from build123d import *

# Parameters (mm, degrees)
SKETCH1_W           = 56.15
SKETCH1_H           = 25.4
BOSS_EXTRUDE1_DEPTH = 2.54
SKETCH2_W           = 56.15
SKETCH2_H           = 25.4
BOSS_EXTRUDE2_DEPTH = 2.54
SKETCH11_W          = 56.15
SKETCH11_H          = 25.4
BOSS_EXTRUDE3_DEPTH = 5.715
SKETCH6_R           = 1.774
CUT_EXTRUDE3_DEPTH  = 9.255
SKETCH13_W          = 56.15
SKETCH13_H          = 31.115
BOSS_EXTRUDE4_DEPTH = 11.938
SKETCH14_W          = 12.7
SKETCH14_H          = 8.89
SKETCH14_W_2        = 33.02
CUT_EXTRUDE4_DEPTH  = 32.115
SKETCH17_W          = 10.43
SKETCH17_H          = 22.86
BOSS_EXTRUDE5_DEPTH = 14.097
SKETCH15_R          = 1.778
CUT_EXTRUDE5_DEPTH  = 38.338


with BuildPart() as part:
    # Sketch1 → Boss-Extrude1 (new body)
    with BuildSketch(Plane(origin=(0, 0, 0), x_dir=(1, 0, 0), z_dir=(0, 1, 0))):
        with Locations((28.075, 12.7)):
            Rectangle(SKETCH1_W, SKETCH1_H)
    extrude(amount=-BOSS_EXTRUDE1_DEPTH)

    # Sketch2 → Boss-Extrude2 (add)
    with BuildSketch(Plane.XY):
        with Locations((28.075, -12.7)):
            Rectangle(SKETCH2_W, SKETCH2_H)
    extrude(amount=-BOSS_EXTRUDE2_DEPTH)

    # Sketch11 → Boss-Extrude3 (add)
    with BuildSketch(Plane(origin=(0, 0, 0), x_dir=(1, 0, 0), z_dir=(0, 1, 0))):
        with Locations((28.075, 12.7)):
            Rectangle(SKETCH11_W, SKETCH11_H)
    extrude(amount=BOSS_EXTRUDE3_DEPTH)

    # Sketch6 → Cut-Extrude3 (cut, through all)
    with BuildSketch(Plane.XZ.offset(2.54)):
        with Locations((52.852, -22.102)):
            Circle(SKETCH6_R)
        with Locations((52.852, -9.664)):
            Circle(SKETCH6_R)
        with Locations((3.298, -9.664)):
            Circle(SKETCH6_R)
        with Locations((3.298, -22.102)):
            Circle(SKETCH6_R)
    extrude(amount=-CUT_EXTRUDE3_DEPTH, mode=Mode.SUBTRACT)

    # Sketch13 → Boss-Extrude4 (add)
    with BuildSketch(Plane.XY):
        with Locations((28.075, -9.8425)):
            Rectangle(SKETCH13_W, SKETCH13_H)
    extrude(amount=BOSS_EXTRUDE4_DEPTH)

    # Sketch14 → Cut-Extrude4 (cut, through all)
    with BuildSketch(Plane.XZ.offset(25.4)):
        with Locations((6.35, 7.493)):
            Rectangle(SKETCH14_W, SKETCH14_H)
        with Locations((39.64, 7.493)):
            Rectangle(SKETCH14_W_2, SKETCH14_H)
    extrude(amount=-CUT_EXTRUDE4_DEPTH, mode=Mode.SUBTRACT)

    # Sketch17 → Boss-Extrude5 (add)
    with BuildSketch(Plane(origin=(0, 0, -2.54), x_dir=(-1, 0, 0), z_dir=(0, 0, -1))):
        with Locations((-17.915, -13.97)):
            Rectangle(SKETCH17_W, SKETCH17_H)
    extrude(amount=BOSS_EXTRUDE5_DEPTH)

    # Sketch15 → Cut-Extrude5 (cut, through all)
    with BuildSketch(Plane.XY.offset(11.938)):
        with Locations((17.825, -12.45)):
            Circle(SKETCH15_R)
    extrude(amount=-CUT_EXTRUDE5_DEPTH, mode=Mode.SUBTRACT)


solid = part.part
Verification items for the finished model (mm, model axes). A direction names the side the tool comes from. Coordinates: 2 decimals unless noted, no trailing zeros. Loops run counter-clockwise (first coordinate to the right, second up) from the corner with the lowest first, then second, coordinate; pieces in that order, holes last. Notation, with made-up numbers: (77, 77.25) -> (127, 77.25) arc R18 ccw to (127, 81.25) -> close; hole circle Ø1 at (76.25, 32.25). An arc over 180 degrees is marked (long way). Write each question's results on one line, items separated by ' | '.
Item 1: Material ranges on L1, parallel to Z at x = 53, y = -1.5; L2, parallel to Z at x = 6.5, y = -7.5; L3, parallel to X at y = -1.5, z = -23, recorded low to high.
Found:
L1: z = -25.4 to -23.87, -20.33 to -11.43, -7.9 to 3.05 | L2: z = -2.54 to 3.05 | L3: x = 0 to 1.77, 4.83 to 51.32, 54.38 to 56.15
Item 2: Mould release check, pull along X, two halves, no side actions. Record for faces 4 (the face through (0, -3, -2)), 5 (the face through (24, -25.4, -2)), 6 (the face through (4.117, 1.53, -23.676)): +X half, -X half, draft (parallel to the pull), parting line (faces both ways), or undercut.
Found:
face 4: -X half | face 5: draft | face 6: undercut
Item 3: Tool access check on faces 1 (the face through (23.13, -10, 7)), 2 (the face through (12.7, -14, -9)), 3 (the face through (39, -14, -2.54)). Record the directions out of +Z, -Z, +X, -X, +Y, -Y that give a thin tool (end or side, any length) a straight path to the whole face; none if there is none.
Found:
face 1: +Z, +X, +Y, -Y | face 2: -Z, -X, -Y | face 3: -Z, +X, -Y
Item 4: Section check B-B, the plane y = -22. Enter the section's corners in (x, z).
Found:
outline: (0, -2.54) -> (12.7, -2.54) -> (12.7, -16.64) -> (23.13, -16.64) -> (23.13, -2.54) -> (56.15, -2.54) -> (56.15, 3.05) -> (23.13, 3.05) -> (23.13, 11.94) -> (12.7, 11.94) -> (12.7, 3.05) -> (0, 3.05) -> close
Item 5: Gauge pin test, flat ends, axial feed: pin 1 (7 mm diameter, centred on y = -13.5, z = -7, fed in from +X); pin 2 (5 mm diameter, centred on x = 19.5, y = -18.5, fed in from -Z); pin 3 (6.5 mm diameter, centred on x = 7, y = -17, fed in from -Z); pin 4 (10 mm diameter, centred on y = -6, z = 5.5, fed in from -X). Record the tip position at first contact, or that the pin passes through.
Found:
pin 1: stops at x = 23.13 | pin 2: stops at z = -16.64 | pin 3: stops at z = -2.54 | pin 4: stops at x = 0
Item 6: Section check D-D, the plane y = -12.45. Enter the section's corners in (x, z), plus the area to 3 significant figures.
Found:
outline: (0, -2.54) -> (12.7, -2.54) -> (12.7, -16.64) -> (16.05, -16.64) -> (16.05, 11.94) -> (12.7, 11.94) -> (12.7, 3.05) -> (0, 3.05) -> close; (19.6, -16.64) -> (23.13, -16.64) -> (23.13, -2.54) -> (56.15, -2.54) -> (56.15, 3.05) -> (23.13, 3.05) -> (23.13, 11.94) -> (19.6, 11.94) -> close | area: 452 mm2
Item 7: Section check A-A, the plane z = -9. Enter the section's corners in (x, y) (3 decimals), plus the area to 3 significant figures.
Found:
outline: (0, -2.54) -> (1.653, -2.54) -> (1.653, 5.715) -> (0, 5.715) -> close; (4.943, -2.54) -> (12.7, -2.54) -> (12.7, -25.4) -> (23.13, -25.4) -> (23.13, -2.54) -> (51.207, -2.54) -> (51.207, 5.715) -> (4.943, 5.715) -> close; (54.497, -2.54) -> (56.15, -2.54) -> (56.15, 5.715) -> (54.497, 5.715) -> close; hole circle Ø3.556 at (17.825, -12.45) | area: 638 mm2
Item 8: Section check C-C, the plane x = 8. Enter the section's corners in (y, z) (3 decimals).
Found:
outline: (-25.4, -2.54) -> (-2.54, -2.54) -> (-2.54, -25.4) -> (5.715, -25.4) -> (5.715, 3.048) -> (-25.4, 3.048) -> close
